Geometry check sheet. Reference: the model listing, model coordinates, mm. Give positions to 0.01 mm unless a question says otherwise; leave off trailing zeros.
(1) Depth check by flat-ended pin: P1, Ø3, axis at y = -6, z = -18.5, coming from the +X side; P2, Ø1.6, axis at y = 0.5, z = 69.5, coming from the +X side; P3, Ø1.6, axis at x = -0.5, z = 64, coming from the +Y side; P4, Ø2, axis at x = -9, y = -3, coming from the +Z side. Enter the tip coordinate at first touch or a pass-through.
(2) Cross-section at A-A (z = 32.5). Count the separate pieces of the cut face and the enclosed holes in it, and give its area (3 significant figures).
(3) Thickness scan on line 1 along Y through (x, z) = (0.25, 63.5); line 2 along X through (y, z) = (2, 72); line 3 along X through (y, z) = (6.5, -18). Record the ranges inside material, lowest first.
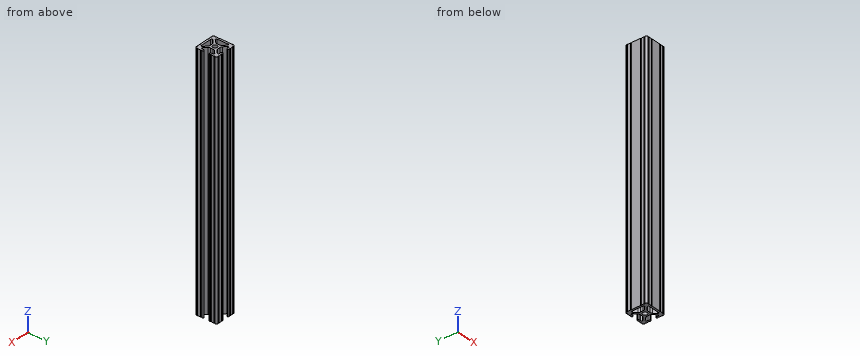
```python
from build123d import *

# Parameters (mm, degrees)
SKETCH3_R                = 2.6035
BOSS_EXTRUDE1_DEPTH      = 142.875
BOSS_EXTRUDE1_DEPTH_BACK = 142.875


with BuildPart() as part:
    # Sketch3 → Boss-Extrude1 (new body, two sides)
    with BuildSketch(Plane.XY) as boss_extrude1_sk:
        with BuildLine():
            Line((6.3331344, -12.7), (9.5504, -12.7))
            ThreePointArc((9.5504, -12.7), (10.058323491, -12.192000006), (10.566399977, -12.699846982))
            ThreePointArc((10.566399977, -12.699846982), (12.082522516, -12.082522516), (12.699846982, -10.566399977))
            ThreePointArc((12.699846982, -10.566399977), (12.192000006, -10.058323491), (12.7, -9.5504))
            Line((12.7, -9.5504), (12.7, -6.3330836))
            ThreePointArc((12.7, -6.3330836), (12.192, -5.8250836), (12.7, -5.3170836))
            Line((12.7, -5.3170836), (12.7, -4.28752))
            ThreePointArc((12.7, -4.28752), (12.392749156, -3.545750844), (11.65098, -3.2385))
            Line((11.65098, -3.2385), (11.53922, -3.2385))
            ThreePointArc((11.53922, -3.2385), (10.797450844, -3.545750844), (10.4902, -4.28752))
            Line((10.4902, -4.28752), (10.4902, -6.402089023))
            ThreePointArc((10.4902, -6.402089023), (9.856394933, -7.351113629), (8.736962546, -7.129240479))
            Line((8.736962546, -7.129240479), (5.440484187, -3.838768792))
            ThreePointArc((5.440484187, -3.838768792), (4.75073678, -2.808015636), (4.5085, -1.591658411))
            Line((4.5085, -1.591658411), (4.5085, 1.591658411))
            ThreePointArc((4.5085, 1.591658411), (4.75073678, 2.808015636), (5.440484187, 3.838768792))
            Line((5.440484187, 3.838768792), (8.736962546, 7.129240479))
            ThreePointArc((8.736962546, 7.129240479), (9.856394933, 7.351113629), (10.4902, 6.402089023))
            Line((10.4902, 6.402089023), (10.4902, 4.28752))
            ThreePointArc((10.4902, 4.28752), (10.797450844, 3.545750844), (11.53922, 3.2385))
            Line((11.53922, 3.2385), (11.65098, 3.2385))
            ThreePointArc((11.65098, 3.2385), (12.392749156, 3.545750844), (12.7, 4.28752))
            Line((12.7, 4.28752), (12.7, 5.3171344))
            ThreePointArc((12.7, 5.3171344), (12.192, 5.8251344), (12.7, 6.3331344))
            Line((12.7, 6.3331344), (12.7, 9.5504))
            ThreePointArc((12.7, 9.5504), (12.192000006, 10.058323491), (12.699846982, 10.566399977))
            ThreePointArc((12.699846982, 10.566399977), (12.082522516, 12.082522516), (10.566399977, 12.699846982))
            ThreePointArc((10.566399977, 12.699846982), (10.058323491, 12.192000006), (9.5504, 12.7))
            Line((9.5504, 12.7), (6.3330836, 12.7))
            ThreePointArc((6.3330836, 12.7), (5.8250836, 12.192), (5.3170836, 12.7))
            Line((5.3170836, 12.7), (4.28752, 12.7))
            ThreePointArc((4.28752, 12.7), (3.545750844, 12.392749156), (3.2385, 11.65098))
            Line((3.2385, 11.65098), (3.2385, 11.53922))
            ThreePointArc((3.2385, 11.53922), (3.545750844, 10.797450844), (4.28752, 10.4902))
            Line((4.28752, 10.4902), (6.476795923, 10.4902))
            ThreePointArc((6.476795923, 10.4902), (7.432175542, 9.851520654), (7.207206853, 8.724555432))
            Line((7.207206853, 8.724555432), (3.900315394, 5.423689619))
            ThreePointArc((3.900315394, 5.423689619), (2.8709819, 4.736928798), (1.657299581, 4.4958))
            Line((1.657299581, 4.4958), (-1.553667902, 4.4958))
            ThreePointArc((-1.553667902, 4.4958), (-2.767350221, 4.736928798), (-3.796683715, 5.423689619))
            Line((-3.796683715, 5.423689619), (-7.134200223, 8.755124678))
            ThreePointArc((-7.134200223, 8.755124678), (-7.355273948, 9.862578342), (-6.416435163, 10.4902))
            Line((-6.416435163, 10.4902), (-4.28752, 10.4902))
            ThreePointArc((-4.28752, 10.4902), (-3.545750844, 10.797450844), (-3.2385, 11.53922))
            Line((-3.2385, 11.53922), (-3.2385, 11.65098))
            ThreePointArc((-3.2385, 11.65098), (-3.545750844, 12.392749156), (-4.28752, 12.7))
            Line((-4.28752, 12.7), (-5.3171344, 12.7))
            ThreePointArc((-5.3171344, 12.7), (-5.8251344, 12.192), (-6.3331344, 12.7))
            Line((-6.3331344, 12.7), (-9.5504, 12.7))
            ThreePointArc((-9.5504, 12.7), (-10.058323491, 12.192000006), (-10.566399977, 12.699846982))
            ThreePointArc((-10.566399977, 12.699846982), (-12.082522516, 12.082522516), (-12.699846982, 10.566399977))
            ThreePointArc((-12.699846982, 10.566399977), (-12.192000006, 10.058323491), (-12.7, 9.5504))
            Line((-12.7, 9.5504), (-12.7, 6.3331344))
            ThreePointArc((-12.7, 6.3331344), (-12.192, 5.8251344), (-12.7, 5.3171344))
            Line((-12.7, 5.3171344), (-12.7, -5.3170836))
            ThreePointArc((-12.7, -5.3170836), (-12.192, -5.8250836), (-12.7, -6.3330836))
            Line((-12.7, -6.3330836), (-12.7, -9.5504))
            ThreePointArc((-12.7, -9.5504), (-12.192000006, -10.058323491), (-12.699846982, -10.566399977))
            ThreePointArc((-12.699846982, -10.566399977), (-12.082522516, -12.082522516), (-10.566399977, -12.699846982))
            ThreePointArc((-10.566399977, -12.699846982), (-10.058323491, -12.192000006), (-9.5504, -12.7))
            Line((-9.5504, -12.7), (-6.3330836, -12.7))
            ThreePointArc((-6.3330836, -12.7), (-5.8250836, -12.192), (-5.3170836, -12.7))
            Line((-5.3170836, -12.7), (5.3171344, -12.7))
            ThreePointArc((5.3171344, -12.7), (5.8251344, -12.192), (6.3331344, -12.7))
        make_face()
        Circle(SKETCH3_R, mode=Mode.SUBTRACT)
        with BuildLine():
            Line((-8.753441447, -7.145689354), (-5.440484187, -3.838768792))
            ThreePointArc((-5.440484187, -3.838768792), (-4.75073678, -2.808015636), (-4.5085, -1.591658411))
            Line((-4.5085, -1.591658411), (-4.5085, 1.591658411))
            ThreePointArc((-4.5085, 1.591658411), (-4.75073678, 2.808015636), (-5.440484187, 3.838768792))
            Line((-5.440484187, 3.838768792), (-8.736962546, 7.129240479))
            ThreePointArc((-8.736962546, 7.129240479), (-9.856394933, 7.351113629), (-10.4902, 6.402089023))
            Line((-10.4902, 6.402089023), (-10.4902, -6.425372487))
            ThreePointArc((-10.4902, -6.425372487), (-9.862352148, -7.36547709), (-8.753441447, -7.145689354))
        make_face(mode=Mode.SUBTRACT)
        with BuildLine():
            Line((7.147805753, -8.66526257), (3.900315394, -5.423689619))
            ThreePointArc((3.900315394, -5.423689619), (2.8709819, -4.736928798), (1.657299581, -4.4958))
            Line((1.657299581, -4.4958), (-1.657299581, -4.4958))
            ThreePointArc((-1.657299581, -4.4958), (-2.8709819, -4.736928798), (-3.900315394, -5.423689619))
            Line((-3.900315394, -5.423689619), (-7.153722341, -8.671168377))
            ThreePointArc((-7.153722341, -8.671168377), (-7.374796065, -9.77862204), (-6.435957281, -10.406243698))
            Line((-6.435957281, -10.406243698), (6.427597582, -10.406243698))
            ThreePointArc((6.427597582, -10.406243698), (7.369631963, -9.776485757), (7.147805753, -8.66526257))
        make_face(mode=Mode.SUBTRACT)
    extrude(amount=BOSS_EXTRUDE1_DEPTH)
    extrude(boss_extrude1_sk.sketch, amount=-BOSS_EXTRUDE1_DEPTH_BACK)


solid = part.part
```
Reply:
1. P1: stops at x = 12.7
1. P2: stops at x = 4.51
1. P3: stops at y = 4.5
1. P4: passes through
2. separate pieces: 1
2. enclosed holes: 3
2. area: 313 mm2
3. line 1: y = -12.7 to -10.41, -4.5 to -2.59, 2.59 to 4.5
3. line 2: x = -12.7 to -10.49, -4.53 to -1.67, 1.67 to 4.53
3. line 3: x = -12.7 to -10.49, -8.11 to -4.87, 4.98 to 8.11, 10.49 to 12.7
